Part print with two shaded views. Sizes in mm from the minimum x, y, z corner. A direction names the side the tool comes from. Round coordinates to 2 decimals unless told otherwise and drop trailing zeros. Write each loop counter-clockwise with the first axis right and the second up, starting at its lowest first coordinate (ties: lowest second). Pieces come first, ordered by that corner, then holes.
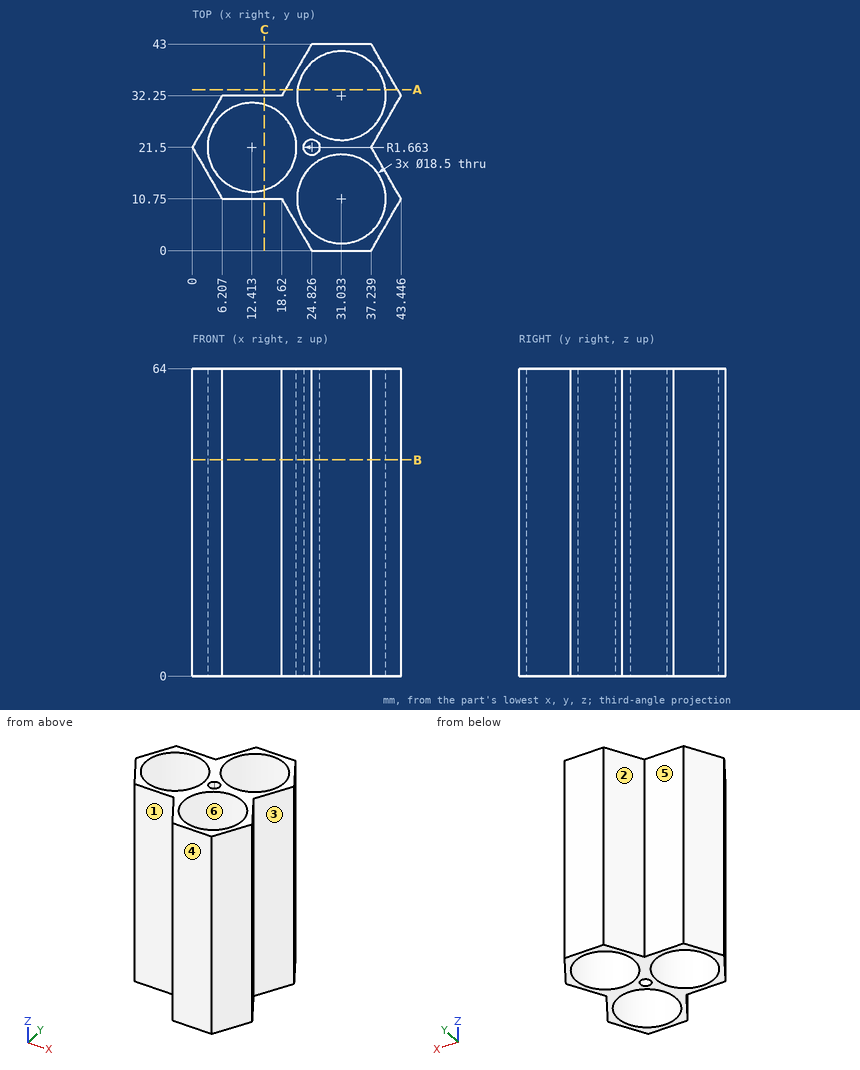
Q1. Mould opens along Y. For the marked faces 4, 5 and 6 say: +Y half, -Y half, draft (parallel to the pull), parting line (faces both ways), or undercut.
Values follow:
face 4: -Y half
face 5: +Y half
face 6: undercut
Q2. Drop flat-ended pins along their axis: pin 1 (2 mm diameter, centred on x = 13, z = 56, fed in from -Y); pin 2 (13.5 mm diameter, centred on x = 14, z = 38.5, fed in from +Y); pin 3 (1.5 mm diameter, centred on y = 27.5, z = 42.5, fed in from +X) (1 decimal). Give the stop position or say it passes through.
Values follow:
pin 1: stops at y = 10.75
pin 2: stops at y = 35.94
pin 3: stops at x = 41.1
Q3. Which spindle directions (+Z, -Z, +X, -X, +Y, -Y) get a long thin tool onto all of the face, cutting with end or side? Do the marked faces 1, 2 and 3. Say none if no direction does.
Values follow:
face 1: +Z, -Z, -X, -Y
face 2: +Z, -Z, -X, +Y
face 3: +Z, -Z, +X
Q4. Cut at A-A on y = 33.5. Write the cut outline in (x, z).
Values follow:
outline: (19.34, 0) - (21.87, 0) - (21.87, 64) - (19.34, 64) - close; (40.2, 0) - (42.72, 0) - (42.72, 64) - (40.2, 64) - close
Q5. Cut at C-C on x = 15. Write the cut outline in (y, z).
Values follow:
outline: (10.75, 0) - (12.62, 0) - (12.62, 64) - (10.75, 64) - close; (30.38, 0) - (32.25, 0) - (32.25, 64) - (30.38, 64) - close
Q6. Wall check: L1, parallel to Y at x = 29, z = 33.5 (1 decimal); L2, parallel to Y at x = 36, z = 45.5 (1 decimal); L3, parallel to Y at x = 19, z = 17.5 (1 decimal). Give the ranges that are in metal, low to high.
Values follow:
L1: y = 0 to 1.7, 19.8 to 23.2, 41.3 to 43
L2: y = 0 to 2.9, 18.6 to 24.4, 40.1 to 43
L3: y = 10.1 to 15, 28 to 32.9
Q7. Cut at B-B on z = 45. State how many separate pieces and enclosed holes the cut face has, plus the area to 3 significant figures.
Values follow:
separate pieces: 1
enclosed holes: 4
area: 386 mm2
